Could you check a few things on this model? Use its own coordinates, in mm. Face numbers are marked on the shaded views. A direction names the side the tool comes from. Round coordinates to 2 decimals unless told otherwise and drop trailing zeros. Write each loop counter-clockwise with the first axis right and the second up, starting at its lowest first coordinate (ties: lowest second). Pieces come first, ordered by that corner, then holes. Notation, with made-up numbers: (54.25, 38.25) - (96.25, 38.25) arc R15 cw to (96.25, 60.25) - close; hole circle Ø7 at (43.5, -4). An arc over 180 degrees is marked (long way). Put each result on its own line as item: value.
from build123d import *

# Parameters (mm, degrees)
F0_R     = 45.9871931788
F1_DEPTH = 12.7
F4_R     = 35.5142998493
F5_DEPTH = 20
F6_SIZE  = 5


# Not quite as in the source:
# - the program builds the solid bodies; features that only make, move or delete a surface that nothing else refers to are left out


with BuildPart() as f1:
    # F0 (on Front) → F1 (new body, symmetric)
    with BuildSketch(Plane.XZ):
        with Locations((0, 5.3770393133)):
            Circle(F0_R)
    extrude(amount=F1_DEPTH, both=True)

    # F4 (on face) → F5 (join)
    with BuildSketch(Plane(origin=(0, 12.7, 0), x_dir=(-1, 0, 0), z_dir=(0, 1, 0))):
        with Locations((0, 5.3770393133)):
            Circle(F4_R)
    extrude(amount=F5_DEPTH)

    # F6
    f6_edges = [f1.edges().sort_by_distance(p)[0] for p in [
        (-45.987193, 12.7, 5.377039),
    ]]
    chamfer(f6_edges, length=F6_SIZE)


solid = f1.part
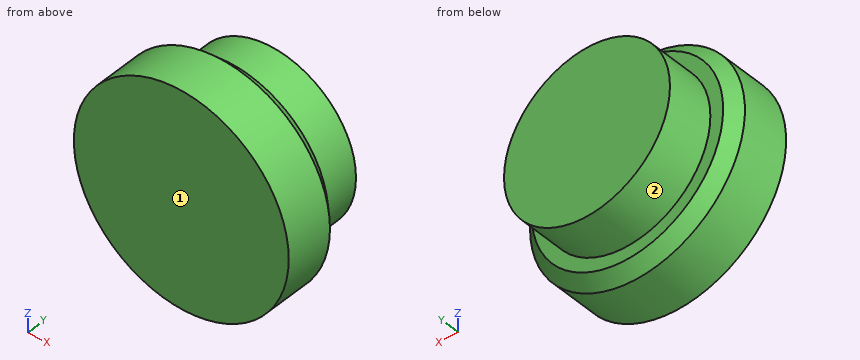
(1) Imagine slicing it at A-A, the plane x = 0. List the corners of the cut face in (y, z) for me, then the cut area to 3 significant figures.
Values found:
outline: (-12.7, -40.61) - (7.7, -40.61) - (12.7, -35.61) - (12.7, -30.14) - (32.7, -30.14) - (32.7, 40.89) - (12.7, 40.89) - (12.7, 46.36) - (7.7, 51.36) - (-12.7, 51.36) - close
area: 3,730 mm^2
(2) Please list where these lines run through material, in increasing order: probe 1 along Z at (x, y) = (-2.5, 17); probe 2 along Z at (x, y) = (-24.5, 18.5); probe 3 along Y at (x, z) = (-14, -31). Write a range as from..to.
Values found:
probe 1: z = -30.05..40.8
probe 2: z = -20.33..31.09
probe 3: y = -12.7..12.7
(3) I'm going to push flat-ended pins straight in: pin 1 (5 mm diameter, centred on x = -18, y = -3.5, fed in from +Z); pin 2 (12 mm diameter, centred on x = 2.5, y = 6, fed in from -Z); pin 3 (2 mm diameter, centred on x = 22.5, y = 25.5, fed in from +Z). Where does each tip first touch, or does it pass through?
Values found:
pin 1: stops at z = 48.67
pin 2: stops at z = -40.61
pin 3: stops at z = 33.64
(4) Imagine slicing it at B-B, the plane y = 29.5. List the corners of the cut face in (x, z) for me, then the cut area to 3 significant figures.
Values found:
outline: circle Ø71.03 at (0, 5.38)
area: 3,960 mm^2
(5) For the marked faces 1 and 2, which set-ups out of +Z, -Z, +X, -X, +Y, -Y let a thin tool reach every point of the face, with its end or its side?
Values found:
face 1: +Z, -Z, +X, -X, -Y
face 2: +Y
